Autodesk Inventor part; units mm, degrees
ref_plane "YZ Plane" through (0, 0, 0) normal (1, 0, 0) x (0, 1, 0)
ref_plane "XZ Plane" through (0, 0, 0) normal (0, 1, 0) x (-1, 0, 0)
ref_plane "XY Plane" through (0, 0, 0) normal (0, 0, 1) x (1, 0, 0)
sketch "草圖1" plane through (0, 0, 0) normal (0, 0, 1) x (1, 0, 0)
  line L0 (0, 0) -> (-46.9602, 0) construction
  line L1 (0, 0) -> (0, 45.4619) construction
  line L2 (-65, -7.5) -> (65, -7.5)
  line L3 (65, -7.5) -> (65, 7.5)
  line L4 (65, 7.5) -> (-65, 7.5)
  line L5 (-65, 7.5) -> (-65, -7.5)
  line L6 (-65, -7.5) -> (65, 7.5) construction
  line L7 (65, -7.5) -> (-65, 7.5) construction
  circle A0 centre (0, 1.5799) radius 5
  dimension "d0" = 15
  dimension "d1" = 130
  dimension "d5" = 10
extrude "擠出1" add sketch "草圖1" along normal mid plane 2.5
fillet "圓角1" radius 5 2 edges at (-65, 7.5, 0) (65, 7.5, 0)
properties part number "0 零件" material "橡膠"
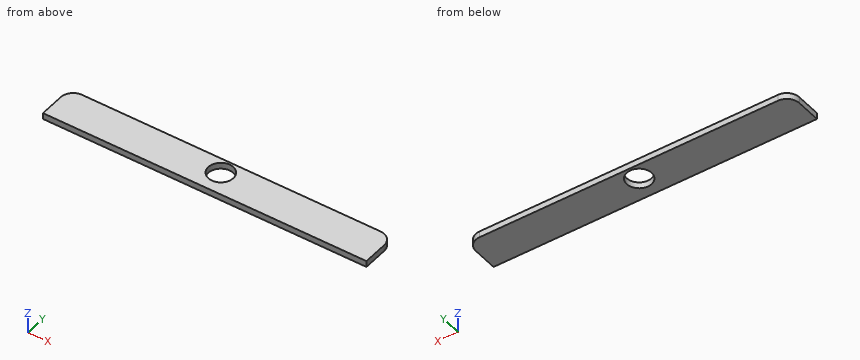
Here's how the part is built. I have some questions about the finished solid (model axes, mm). Round coordinates to 2 decimals unless told otherwise and drop trailing zeros. Order: outer loops, then holes, each group sorted by start corner. A loop starts at its lowest first (then second) coordinate and runs counter-clockwise, first axis right, second up. Notation, with made-up numbers: M -16,0.25 L -2,0.25 A33 ccw -2,33.25 Z; hole C -14.75,-19 d9. An arc over 180 degrees is marked long. Use CSV: the item, a comma, the result in double quotes.
1) I want a section at A-A (x = 0). List the corners of the cut face in (y, z) for me, then the cut area to 3 significant figures.
Taken from the geometry:
outline,"M -7.5,-1.25 L -3.42,-1.25 L -3.42,1.25 L -7.5,1.25 Z; M 6.58,-1.25 L 7.5,-1.25 L 7.5,1.25 L 6.58,1.25 Z"
area,"12.5 mm^2"
2) I want a section at B-B (z = 0.65). List the corners of the cut face in (x, y) for me, then the cut area to 3 significant figures.
Taken from the geometry:
outline,"M -65,-7.5 L 65,-7.5 L 65,2.5 A5 ccw 60,7.5 L -60,7.5 A5 ccw -65,2.5 Z; hole C 0,1.58 d10"
area,"1,860 mm^2"
3) I need wall thicknesses on line 1 along Y through (x, z) = (0, 0.7); line 2 along X through (y, z) = (1.5, -0.4); line 3 along X through (y, z) = (0.5, 0). Which ranges of each line are inside material? Lowest first, please. Write a range as [from, to].
Taken from the geometry:
line 1,"[-7.5, -3.42], [6.58, 7.5]"
line 2,"[-65, -5], [5, 65]"
line 3,"[-65, -4.88], [4.88, 65]"
